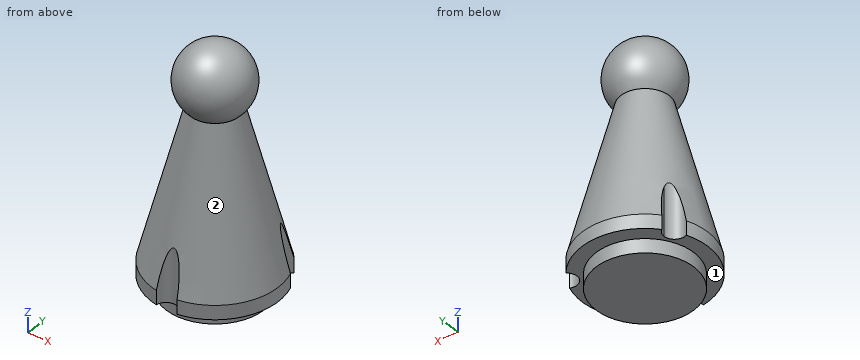
from build123d import *

# Parameters (mm, degrees)
F0_R      = 7
F1_DEPTH  = 2
F2_R      = 9
F3_DEPTH  = 2
F3_FACE_R = 9
F5_R      = 2.5
F10_DEPTH = 32.001


with BuildPart() as f1:
    # F0 (on Top) → F1 (new body)
    with BuildSketch(Plane.XY):
        Circle(F0_R)
    extrude(amount=F1_DEPTH)

    # F2 (on face) → F3 (join)
    with BuildSketch(Plane.XY.offset(2)):
        Circle(F2_R)
    extrude(amount=F3_DEPTH)

    # F3_face (on face) → F6 section 0
    with BuildSketch(Plane.XY.offset(4)):
        Circle(F3_FACE_R)
    # F5 (on offset) → F6 section 1
    with BuildSketch(Plane.XY.offset(29)):
        Circle(F5_R)
    loft()

    # F7 (on face) → F8 (revolve)
    with BuildSketch(Plane.XY.offset(29)):
        with BuildLine():
            ThreePointArc((-5, 0), (0, -5), (5, 0))
            Line((5, 0), (2.5, 0))
            ThreePointArc((2.5, 0), (0, -2.5), (-2.5, 0))
            Line((-2.5, 0), (-5, 0))
        make_face()
    revolve(axis=Axis((0, 0, 29), (1, 0, 0)))

    # F9 (on face) → F10 (cut, through all)
    with BuildSketch(Plane(origin=(0, 0, 2), x_dir=(1, 0, 0), z_dir=(0, 0, -1))):
        with BuildLine():
            ThreePointArc((1.4947825929, 8.875), (0, 9), (-1.4947825929, 8.875))
            ThreePointArc((-1.4947825929, 8.875), (0, 7.5), (1.4947825929, 8.875))
        make_face()
        with BuildLine():
            ThreePointArc((-6.2942286341, -4.5), (-6.9907073778, -3.2333691972), (-8.433366755, -3.1429803014))
            ThreePointArc((-8.433366755, -3.1429803014), (-7.7942286341, -4.5), (-6.9385841621, -5.7320196986))
            ThreePointArc((-6.9385841621, -5.7320196986), (-6.4650434122, -5.1951738244), (-6.2942286341, -4.5))
        make_face()
        with BuildLine():
            ThreePointArc((6.9385841621, -5.7320196986), (7.7942286341, -4.5), (8.433366755, -3.1429803014))
            ThreePointArc((8.433366755, -3.1429803014), (6.4951905284, -3.75), (6.9385841621, -5.7320196986))
        make_face()
    extrude(amount=-F10_DEPTH, mode=Mode.SUBTRACT)


solid = f1.part
The listing builds one solid part. Answer for the finished solid, in the listing's coordinates (mm). Face numbers are marked on the shaded views. Coordinates: 2 decimals unless noted, no trailing zeros. Order: outer loops, then holes, each group sorted by start corner. A loop starts at its lowest first (then second) coordinate and runs counter-clockwise, first axis right, second up.
Q1. A cutting plane is placed at D-D, the plane z = 12. Write down the section's boundary in (x, y), and give its area (3 significant figures).
Q2. Consider line 1 (Z direction, x = -1.5, y = 0.25); line 2 (Z direction, x = 0.5, y = 1); line 3 (X direction, y = -6.25, z = 10). Determine where each line is inside the solid, lowest interval first.
Q3. A cutting plane is placed at C-C, the plane z = 30. Write down the section's boundary in (x, y).
Q4. For a pull along Z with two mould halves and no side action, classify the marked faces 1 and 2 as pulls with the +Z half, pulls with the -Z half, needs draft (parallel to the pull), parting line crosses it, or undercut.
Q5. Given P1, Ø5, axis at x = 3, y = 1, coming from the +Z side; P2, Ø6, axis at x = 2.5, z = 17.5, coming from the +Y side; P3, Ø6, axis at y = -3, z = 26, coming from the -X side, each flat-ended and moving along its own axis, determine where each tip first touches the part or whether it passes through.
Q6. A cutting plane is placed at B-B, the plane z = 18.5. Write down the section's boundary in (x, y).
Q7. A cutting plane is placed at A-A, the plane x = 0. Write down the section's boundary in (y, z).
Answers follow:
1. outline: circle Ø13.84 at (0, 0)
1. area: 150 mm2
2. line 1: z = 0 to 29, 30.98 to 33.76
2. line 2: z = 0 to 29, 31.24 to 33.87
2. line 3: x = -4.04 to 4.04
3. outline: circle Ø9.8 at (0, 0); hole circle Ø4.58 at (0, 0)
4. face 1: pulls with the -Z half
4. face 2: undercut
5. P1: stops at z = 33.96
5. P2: stops at y = 6.08
5. P3: stops at x = -4.84
6. outline: circle Ø10.46 at (0, 0)
7. outline: (-7.5, 2) - (-7, 2) - (-7, 0) - (7, 0) - (7, 2) - (9, 2) - (9, 4) - (3.44, 25.37) arc R5 ccw (long way) to (-3.44, 25.37) - (-7.5, 9.77) - close; hole (-2.5, 29) - (2.5, 29) arc R2.5 ccw to start
